Autodesk Fusion 360 part; units mm, degrees
sketch "Sketch1" plane through (0, 0, 0) normal (0, 0, 1) x (1, 0, 0)
  line L0 (-27.9, 64) -> (27.9, 64)
  line L1 (27.9, 64) -> (27.9, -64)
  line L2 (27.9, -64) -> (-27.9, -64)
  line L3 (-27.9, -64) -> (-27.9, 64)
  line L4 (0, 76.2027) -> (0, 75)
  line L5 (0, 75) -> (0, -75) construction
  line L6 (-56.392, 0) -> (-53.853, 0)
  line L7 (-53.853, 0) -> (53.853, 0) construction
  point P0 (0, 64)
  point P1 (-27.9, 0)
  dimension "d44" = 150
  dimension "d45" = 128
  dimension "d46" = 55.8
extrude "Extrude1" add sketch "Sketch1" along normal blind 7
sketch "Sketch2" plane through (0, -64, 0) normal (0, -1, 0) x (1, 0, 0)
  line L0 (-27.9, 0) -> (27.9, 0)
  line L1 (27.9, 0) -> (27.9, 7)
  line L2 (27.9, 7) -> (-27.9, 7)
  line L3 (-27.9, 7) -> (-27.9, 0)
  line L4 (-27.9, 1.153) -> (-24.9009, 3.6695)
  line L5 (-24.9009, 3.6695) -> (-24.9009, 7)
  line L6 (27.9, 1.153) -> (24.9009, 3.6695)
  line L7 (24.9009, 3.6695) -> (24.9009, 7)
  dimension "d49" = 1.153
  dimension "d50" = 3.915
  dimension "d51" = 40
  dimension "d52" = 1.153
  dimension "d54" = 3.915
  dimension "d55" = 40
extrude "Extrude2" cut sketch "Sketch2" against normal through all contours L2 L3 L4 L5 | L1 L2 L6 L7
sketch "Sketch3" plane through (0, 0, 0) normal (0, 0, -1) x (1, 0, 0)
  line L0 (27.9, 64) -> (-27.9, 64)
  line L1 (-27.9, 64) -> (-27.9, -64)
  line L2 (-27.9, -64) -> (27.9, -64)
  line L3 (27.9, -64) -> (27.9, 64)
  line L4 (0, 64) -> (0, -64) construction
  circle A0 centre (0, 54) radius 1.425
  dimension "d57" = 2.85
  dimension "d58" = 10
extrude "Extrude3" cut sketch "Sketch3" against normal blind 7 contours A0
pattern_linear "R-Pattern1" count 1 spacing 0 along (-1, 0, 0) count 6 spacing 20 along (0, 1, 0) of "Extrude3"
equation "d52 = d49"
equation "d54 = d50"
equation "d55 = d51"
Build history of the part. All positions in model axes, mm. A direction names the side the tool comes from. Round coordinates to 2 decimals unless told otherwise and drop trailing zeros. Write each loop counter-clockwise with the first axis right and the second up, starting at its lowest first coordinate (ties: lowest second). Pieces come first, ordered by that corner, then holes. Notation, with made-up numbers: (64.5, 47) -> (122.5, 47) arc R13 ccw to (122.5, 53) -> close; hole circle Ø9 at (89, 89.25). An arc over 180 degrees is marked (long way). Write item = value, one per line.
(1) Flat gauge pins, fed straight in: pin 1 (2.5 mm diameter, centred on y = 10.5, z = 6, fed in from -X); pin 2 (4 mm diameter, centred on y = -22.5, z = 3.5, fed in from +X); pin 3 (1 mm diameter, centred on y = 6, z = 5, fed in from +X). Where does each tip first touch, or does it go through?
Answer:
pin_1 = -24.9
pin_2 = 27.49
pin_3 = 24.9
(2) Two-plate mould, pull along Y, no slides. Class faces 1 (the face through (0, 64, 3)), 2 (the face through (0.658, -52.736, 3.451)), 3 (the face through (-24.901, -1, 5)): pulls with the +Y half, pulls with the -Y half, needs draft (parallel to the pull), parting line crosses it, or undercut.
Answer:
face_1 = pulls with the +Y half
face_2 = undercut
face_3 = needs draft
(3) Band-saw the part on B-B (z = 5.75). Give the cut face in (x, y) (3 decimals), then the cut area to 3 significant figures.
Answer:
outline = (-24.901, -64) -> (24.901, -64) -> (24.901, 64) -> (-24.901, 64) -> close; hole circle Ø2.85 at (0, -54); hole circle Ø2.85 at (0, -34); hole circle Ø2.85 at (0, -14); hole circle Ø2.85 at (0, 6); hole circle Ø2.85 at (0, 26); hole circle Ø2.85 at (0, 46)
area = 6,340 mm2
(4) Tool access for faces 4 (the face through (-0.31, -12.61, 3.45)), 5 (the face through (24.901, -1, 5)): list every direction of +Z, -Z, +X, -X, +Y, -Y with a clear straight run to the whole face (end or side of a thin tool).
Answer:
face_4 = +Z, -Z
face_5 = +Z, +X, +Y, -Y
(5) Band-saw the part on D-D (y = -38). Give the cut face in (x, z), then the cut area to 3 significant figures.
Answer:
outline = (-27.9, 0) -> (27.9, 0) -> (27.9, 1.15) -> (24.9, 3.67) -> (24.9, 7) -> (-24.9, 7) -> (-24.9, 3.67) -> (-27.9, 1.15) -> close
area = 363 mm2
(6) Band-saw the part on C-C (x = 0). Give the cut face in (y, z) (3 decimals).
Answer:
outline = (-64, 0) -> (-55.425, 0) -> (-55.425, 7) -> (-64, 7) -> close; (-52.575, 0) -> (-35.425, 0) -> (-35.425, 7) -> (-52.575, 7) -> close; (-32.575, 0) -> (-15.425, 0) -> (-15.425, 7) -> (-32.575, 7) -> close; (-12.575, 0) -> (4.575, 0) -> (4.575, 7) -> (-12.575, 7) -> close; (7.425, 0) -> (24.575, 0) -> (24.575, 7) -> (7.425, 7) -> close; (27.425, 0) -> (44.575, 0) -> (44.575, 7) -> (27.425, 7) -> close; (47.425, 0) -> (64, 0) -> (64, 7) -> (47.425, 7) -> close
(7) Band-saw the part on A-A (y = 26). Give the cut face in (x, z) (1 decimal).
Answer:
outline = (-27.9, 0) -> (-1.4, 0) -> (-1.4, 7) -> (-24.9, 7) -> (-24.9, 3.7) -> (-27.9, 1.2) -> close; (1.4, 0) -> (27.9, 0) -> (27.9, 1.2) -> (24.9, 3.7) -> (24.9, 7) -> (1.4, 7) -> close
(8) Probe L1, parallel to X at y = 46, z = 5.75 (3 decimals); L2, parallel to X at y = 1, z = 4.5; L3, parallel to X at y = 13, z = 2.75. List the from-to ranges inside material, lowest first.
Answer:
L1 = -24.901 to -1.425, 1.425 to 24.901
L2 = -24.9 to 24.9
L3 = -26 to 26
